Autodesk Inventor part; units mm, degrees
ref_plane "dia1_XY" through (0, 3.175, 0) normal (1, 0, 0) x (0, 0, -1)
ref_plane "dia1_YZ" through (0, 3.175, 0) normal (0, 0, -1) x (0, 1, 0)
ref_plane "dia1_ZX" through (0, 3.175, 0) normal (0, 1, 0) x (1, 0, 0)
sketch "Sketch_1" plane through (0, 0, 0) normal (0, 0, 1) x (1, 0, 0)
  line L0 (138.1252, 0) -> (0, 0)
  line L1 (0, 0) -> (0, 3.175)
  line L2 (0, 3.175) -> (116.6876, 3.175)
  line L3 (116.6876, 3.175) -> (116.6876, 9.6203)
  line L4 (116.6876, 9.6203) -> (138.1252, 9.6203)
  line L5 (138.1252, 9.6203) -> (138.1252, 0)
  line L6 (138.1252, 0) -> (0, 0)
revolve "Revolution1" add sketch "Sketch_1" angle 360 about axis through (138.1252, 0, 0) along (1, 0, 0)
sketch "Sketch_3" plane through (0, 0, 0) normal (0, 0, 1) x (1, 0, 0)
  line L0 (0, 0) -> (-12.7, 0)
  line L1 (-12.7, 0) -> (-12.7, 2.634)
  line L2 (-12.7, 2.634) -> (-12.159, 3.175)
  line L3 (-12.159, 3.175) -> (0, 3.175)
  line L4 (0, 3.175) -> (0, 0)
  line L5 (0, 0) -> (-12.7, 0)
revolve "Revolution2" add sketch "Sketch_3" angle 360 about axis through (0, 0, 0) along (1, 0, 0)
thread "Thread1"
sketch "Sketch_30" plane through (0, 0, 0) normal (0, 0, 1) x (1, 0, 0)
  line L0 (0, 0) -> (-0.254, 0)
  line L1 (-0.254, 2.921) -> (0, 2.921)
  line L2 (0, 2.921) -> (0, 3.429)
  line L3 (0, 3.429) -> (-0.254, 3.429)
  line L4 (-0.254, 3.429) -> (-0.254, 2.921)
revolve "Revolution3" cut sketch "Sketch_30" angle 360 about axis through (0, 0, 0) along (1, 0, 0)
ref_plane "dia1_XY" through (0, 3.175, 0) normal (1, 0, 0) x (0, 0, -1)
ref_plane "dia1_YZ" through (0, 3.175, 0) normal (0, 0, -1) x (0, 1, 0)
ref_plane "dia1_ZX" through (0, 3.175, 0) normal (0, 1, 0) x (1, 0, 0)
ref_plane "dia12_XY" through (0, 0, 10.9537) normal (1, 0, 0) x (0, 0, -1)
ref_plane "dia12_YZ" through (0, 0, 10.9537) normal (0, 0, -1) x (0, 1, 0)
ref_plane "dia12_ZX" through (0, 0, 10.9537) normal (0, 1, 0) x (1, 0, 0)
ref_plane "dia2_XY" through (0, -3.175, 0) normal (1, 0, 0) x (0, 0, -1)
ref_plane "dia2_YZ" through (0, -3.175, 0) normal (0, 0, -1) x (0, 1, 0)
ref_plane "dia2_ZX" through (0, -3.175, 0) normal (0, 1, 0) x (1, 0, 0)
ref_plane "dia22_XY" through (0, 0, -10.9537) normal (1, 0, 0) x (0, 0, -1)
ref_plane "dia22_YZ" through (0, 0, -10.9537) normal (0, 0, -1) x (0, 1, 0)
ref_plane "dia22_ZX" through (0, 0, -10.9537) normal (0, 1, 0) x (1, 0, 0)
ref_plane "rl1_XY" through (-12.7, 0, 0) normal (1, 0, 0) x (0, 0, -1)
ref_plane "rl1_YZ" through (-12.7, 0, 0) normal (0, 0, -1) x (0, 1, 0)
ref_plane "rl1_ZX" through (-12.7, 0, 0) normal (0, 1, 0) x (1, 0, 0)
ref_plane "rl2_XY" through (0, 0, 0) normal (1, 0, 0) x (0, 0, -1)
ref_plane "rl2_YZ" through (0, 0, 0) normal (0, 0, -1) x (0, 1, 0)
ref_plane "rl2_ZX" through (0, 0, 0) normal (0, 1, 0) x (1, 0, 0)
ref_plane "rod_cp_XY" through (0, 0, 0) normal (1, 0, 0) x (0, 0, -1)
ref_plane "rod_cp_YZ" through (0, 0, 0) normal (0, 0, -1) x (0, 1, 0)
ref_plane "rod_cp_ZX" through (0, 0, 0) normal (0, 1, 0) x (1, 0, 0)
ref_plane "thd1_XY" through (-12.7, 3.175, 0) normal (1, 0, 0) x (0, 0, -1)
ref_plane "thd1_YZ" through (-12.7, 3.175, 0) normal (0, 0, -1) x (0, 1, 0)
ref_plane "thd1_ZX" through (-12.7, 3.175, 0) normal (0, 1, 0) x (1, 0, 0)
ref_plane "thd2_XY" through (-12.7, -3.175, 0) normal (1, 0, 0) x (0, 0, -1)
ref_plane "thd2_YZ" through (-12.7, -3.175, 0) normal (0, 0, -1) x (0, 1, 0)
ref_plane "thd2_ZX" through (-12.7, -3.175, 0) normal (0, 1, 0) x (1, 0, 0)
ref_plane "to_rod_clevis_XY" through (-16.764, 0, 0) normal (1, 0, 0) x (0, 0, -1)
ref_plane "to_rod_clevis_YZ" through (-16.764, 0, 0) normal (0, 0, -1) x (0, 1, 0)
ref_plane "to_rod_clevis_ZX" through (-16.764, 0, 0) normal (0, 1, 0) x (1, 0, 0)
properties part number "C-043-DP0_rod"
Here's how the part is built. I have some questions about the finished solid (model axes, mm). A direction names the side the tool comes from. Coordinates: 2 decimals unless noted, no trailing zeros. Order: outer loops, then holes, each group sorted by start corner. A loop starts at its lowest first (then second) coordinate and runs counter-clockwise, first axis right, second up. Notation, with made-up numbers: (10.5, 2.25) -> (60.5, 2.25) arc R28 cw to (60.5, 33.25) -> close; hole circle Ø3 at (28.5, -6.75). An arc over 180 degrees is marked (long way). Return JSON: item names as keys, results as strings.
1) If we section it at C-C on x = 122: List the corners of the cut face in (y, z) for me, plus the area to 3 significant figures.
Conclusion:
{"outline": "circle Ø19.24 at (0, 0)", "area": "291 mm²"}
2) If I drill on probe 1 along X at (y, z) = (-7, -6.5); probe 2 along Z at (x, y) = (58.5, 0.25); probe 3 along Z at (x, y) = (121, -7.25), over which ranges is the centre line in solid material (lowest first)?
Conclusion:
{"probe 1": "x = 116.69 to 138.13", "probe 2": "z = -3.17 to 3.17", "probe 3": "z = -6.32 to 6.32"}
3) If we section it at D-D on x = 68: List the corners of the cut face in (y, z) for me (3 decimals), plus the area to 3 significant figures.
Conclusion:
{"outline": "circle Ø6.35 at (0, 0)", "area": "31.7 mm²"}
4) If we section it at A-A on y = 0: List the corners of the cut face in (x, z) for me (3 decimals), plus the area to 3 significant figures.
Conclusion:
{"outline": "(-12.7, -2.634) -> (-12.159, -3.175) -> (-0.254, -3.175) -> (-0.254, -2.921) -> (0, -2.921) -> (0, -3.175) -> (116.688, -3.175) -> (116.688, -9.62) -> (138.125, -9.62) -> (138.125, 9.62) -> (116.688, 9.62) -> (116.688, 3.175) -> (0, 3.175) -> (0, 2.921) -> (-0.254, 2.921) -> (-0.254, 3.175) -> (-12.159, 3.175) -> (-12.7, 2.634) -> close", "area": "1,230 mm²"}
5) I'm going to push flat-ended pins straight in: P1, Ø6, axis at x = 47.5, z = 3.5, coming from the -Y side; P2, Ø3, axis at x = 29.5, y = 5.5, coming from the -Z side; P3, Ø8, axis at y = 3, z = -1.5, coming from the -X side; P4, Ø10, axis at x = 40.5, z = 4, coming from the +Y side (3 decimals). Where does each tip first touch, or does it pass through?
Conclusion:
{"P1": "stops at y = -3.14", "P2": "passes through", "P3": "stops at x = -12.7", "P4": "stops at y = 3.175"}
6) On a 3-axis mill with a long thin cutter (end or side, diameter ignored), from which of +Z, -Z, +X, -X, +Y, -Y can I reach the whole of each face in a straight line? I mean faces 1 (the flat face through (-12.7, 0, 0)), 2 (the cylindrical face through (-6.12, -0.69, -3.1)). Say none if no direction works.
Conclusion:
{"face 1": "+Z, -Z, -X, +Y, -Y", "face 2": "-X"}
